```python
from build123d import *

# Parameters (mm, degrees)
F0_R     = 47.5
F2_R     = 35
F4_R     = 52.5
F4_R_2   = 47.5
F5_DEPTH = 10
F6_R     = 5
F6_R_2   = 4
F7_DEPTH = 50


with BuildPart() as f3:
    # F0 (on Top) → F3 section 0
    with BuildSketch(Plane.XY):
        Circle(F0_R)
    # F2 (on offset) → F3 section 1
    with BuildSketch(Plane.XY.offset(-220)):
        Circle(F2_R)
    loft()

    # F4 (on face) → F5 (join)
    with BuildSketch(Plane.XY):
        Circle(F4_R)
        Circle(F4_R_2, mode=Mode.SUBTRACT)
        Circle(F4_R_2)
    extrude(amount=F5_DEPTH)

    # F6 (on face) → F7 (join)
    with BuildSketch(Plane.XY.offset(10)):
        Circle(F6_R)
        Circle(F6_R_2, mode=Mode.SUBTRACT)
    extrude(amount=F7_DEPTH)


solid = f3.part
```
Here's how the part is built. I have some questions about the finished solid (model axes, mm). A direction names the side the tool comes from. Coordinates: 2 decimals unless noted, no trailing zeros. Order: outer loops, then holes, each group sorted by start corner. A loop starts at its lowest first (then second) coordinate and runs counter-clockwise, first axis right, second up. Notation, with made-up numbers: M 19,64 L 49,64 A27 cw 49,99 Z; hole C -14,-38 d10. An arc over 180 degrees is marked long. Answer as a JSON object with one key per item and string values. Group by question number.
(1) Suppose I cut it at C-C, the plane z = -57. Please give me the cut outline in (x, y).
(2) Suppose I cut it at B-B, the plane z = -151.5. Please give me the cut outline in (x, y), then the cut area to 3 significant figures.
(3) I need wall thicknesses on probe 1 along Y at (x, z) = (0, 27); probe 2 along Z at (x, y) = (45, -17); probe 3 along Z at (x, y) = (19.5, 4). Which ranges of each line are inside material? Lowest first, please.
(4) For pin 1 (2.5 mm diameter, centred on x = -2, y = 0, fed in from +Z); pin 2 (1 mm diameter, centred on x = -9.5, z = -114, fed in from +Y); pin 3 (10 mm diameter, centred on y = -9, z = -7.5, fed in from -X), each with a flat end and sliding along its axis, tell me the tip position at first contact or that it passes through.
(5) Suppose I cut it at A-A, the plane x = 0. Please give me the cut outline in (y, z).
(6) Which directions (+Z, -Z, +X, -X, +Y, -Y) give clear straight access to the entire face, cutting with the end or side of a thin tool? Please do faces 1 (the face through (50.076, 15.77, 4.93)), 2 (the face through (-11.9, -46.4, 0)).
(7) If we mould it in two halves opening along X, with no side actions, what happens to faces 3 (the face through (-1.08, -4.88, 34.65)), 4 (the face through (0, 0, -220)), 5 (the face through (0, 0, 10)), 6 (the face through (-0.867, -3.905, 34.65))? For each: released by +X, released by -X, zero draft, split by the parting line, or undercut.
Values found:
{
 "1": {"outline": "C 0,0 d88.52"},
 "2": {"outline": "C 0,0 d77.78", "area": "4,750 mm^2"},
 "3": {"probe 1": "y = -5 to -4, 4 to 5", "probe 2": "z = 0 to 10", "probe 3": "z = -220 to 10"},
 "4": {"pin 1": "stops at z = 10", "pin 2": "stops at y = 40.03", "pin 3": "stops at x = -46.98"},
 "5": {"outline": "M -52.5,0 L -47.5,0 L -35,-220 L 35,-220 L 47.5,0 L 52.5,0 L 52.5,10 L 5,10 L 5,60 L 4,60 L 4,10 L -4,10 L -4,60 L -5,60 L -5,10 L -52.5,10 Z"},
 "6": {"face 1": "+Z, -Z", "face 2": "-Z"},
 "7": {"face 3": "split by the parting line", "face 4": "zero draft", "face 5": "undercut", "face 6": "undercut"}
}
